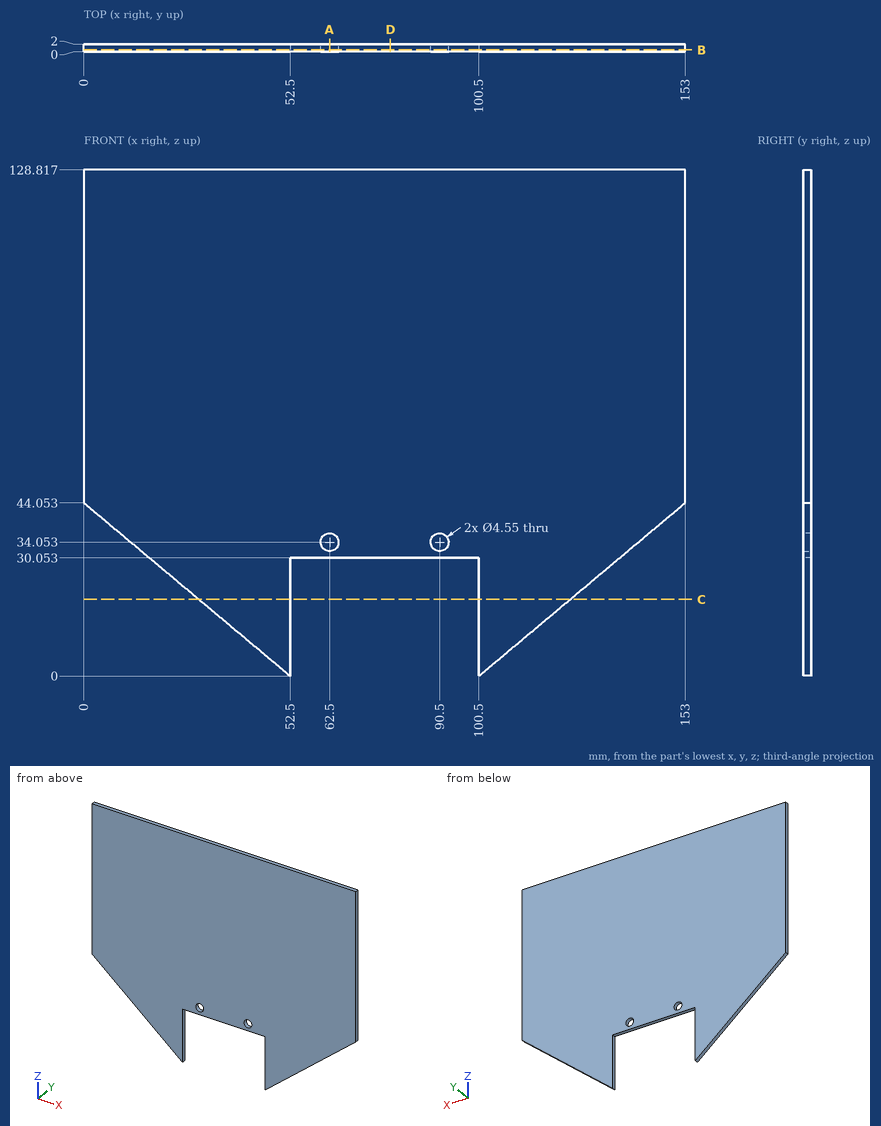
Answer from the drawing. Dimensions are ordinates in mm from the lowest x, y and z of the part. Coordinates: 2 decimals unless noted, no trailing zeros. Order: outer loops, then holes, each group sorted by start corner. A loop starts at its lowest first (then second) coordinate and runs counter-clockwise, first axis right, second up. Notation, with made-up numbers: M -34,73 L 1,73 A23 ccw 1,96 Z; hole C 76,-19 d8. An arc over 180 degrees is marked long. Put each result on its own line as item: value. Start each with the question number.
Item 1: Given pin 1 Ø10 at (x, z) = (137, 45) entering from -Y, flat-ended and moving along its own axis, determine where the tip first touches the part or whether it passes through.
Item 2: Consider probe 1 along X at (y, z) = (1.2, 36) (1 decimal); probe 2 along X at (y, z) = (1.15, 29); probe 3 along X at (y, z) = (0.95, 25.5). Determine where each line is inside the solid, lowest interval first. Write a range as [from, to].
Item 3: Section B-B, the plane y = 0.5 is taken. Count the separate pieces of the cut face and the enclosed holes in it, plus the area to 3 significant figures.
Item 4: Section D-D, the plane x = 78 is taken. Determine the outline of the cut face in (y, z).
Item 5: Section C-C, the plane z = 19.5 is taken. Determine the outline of the cut face in (x, y).
Item 6: Section A-A, the plane x = 62.5 is taken. Determine the outline of the cut face in (y, z).
Computed:
1. pin 1: stops at y = 0
2. probe 1: x = [9.6, 61.3], [63.7, 89.3], [91.7, 143.4]
2. probe 2: x = [17.94, 52.5], [100.5, 135.06]
2. probe 3: x = [22.11, 52.5], [100.5, 130.89]
3. separate pieces: 1
3. enclosed holes: 2
3. area: 15,900 mm2
4. outline: M 0,30.05 L 2,30.05 L 2,128.82 L 0,128.82 Z
5. outline: M 29.26,0 L 52.5,0 L 52.5,2 L 29.26,2 Z; M 100.5,0 L 123.74,0 L 123.74,2 L 100.5,2 Z
6. outline: M 0,30.05 L 2,30.05 L 2,31.78 L 0,31.78 Z; M 0,36.33 L 2,36.33 L 2,128.82 L 0,128.82 Z
